Read the model definition and answer for the solid it produces. Units are mm, in the model's axes. Face numbers are marked on the shaded views. A direction names the side the tool comes from. Coordinates: 2 decimals unless noted, no trailing zeros. Loops run counter-clockwise (first coordinate to the right, second up) from the corner with the lowest first, then second, coordinate; pieces in that order, holes last.
Q1. Section D-D (z = 68) is taken. Give the vertices of the cut face in (x, y), then the cut area to 3 significant figures.
Q2. The mould has two halves that part along X. Classify the marked faces 1, 2, 3 and 4: pulls with the +X half, pulls with the -X half, needs draft (parallel to the pull), parting line crosses it, or undercut.
Q3. Section A-A (z = -12) is taken. Give the vertices of the cut face in (x, y).
Q4. Straight lines are drawn through the part: line 1 (X direction, y = 79, z = 135.5); line 2 (Y direction, x = 197.5, z = 175.5); line 3 (X direction, y = 161, z = 106). For each, find the intervals that lie inside material, in ascending order.
Q5. Section C-C (x = 156) is taken. Give the vertices of the cut face in (y, z).
Q6. Section B-B (y = 369) is taken. Give the vertices of the cut face in (x, z).
Q7. Which of the six approach directions +Z, -Z, +X, -X, +Y, -Y give full straight-line access (tool end or side, diameter ignored) to the marked faces 5, 6 and 7?
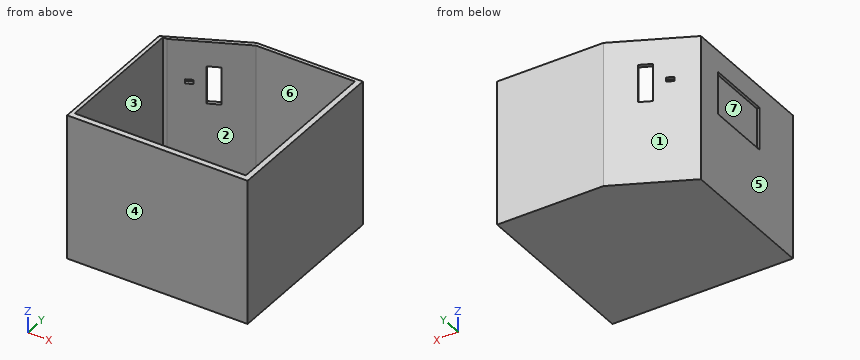
from build123d import *

# Parameters (mm, degrees)
SKETCH1_W           = 508
SKETCH1_H           = 408
SKETCH1_W_2         = 500
SKETCH1_H_2         = 400
BOSS_EXTRUDE1_DEPTH = 500
SKETCH1_3_W         = 500
SKETCH1_3_H         = 400
BOSS_EXTRUDE2_DEPTH = 500
SKETCH2_W           = 120
SKETCH2_H           = 180
CUT_EXTRUDE1_DEPTH  = 7.5
SKETCH4_W           = 481.787571452
SKETCH4_H           = 382.410311639
CUT_EXTRUDE3_DEPTH  = 404
CUT_EXTRUDE4_DEPTH  = 434
CUT_EXTRUDE5_DEPTH  = 404
SKETCH10_W          = 20
SKETCH10_H          = 12
SKETCH10_W_2        = 35.5
SKETCH10_H_2        = 106
CUT_EXTRUDE6_DEPTH  = 24


with BuildPart() as part:
    # Sketch1 → Boss-Extrude1 (new body)
    with BuildSketch(Plane(origin=(0, 0, 0), x_dir=(1, 0, 0), z_dir=(0, 1, 0))):
        with Locations((-0.117405467, -0.781547842)):
            Rectangle(SKETCH1_W, SKETCH1_H)
        with Locations((-0.117405467, -0.781547842)):
            Rectangle(SKETCH1_W_2, SKETCH1_H_2, mode=Mode.SUBTRACT)
    extrude(amount=BOSS_EXTRUDE1_DEPTH)

    # Sketch1_3 → Boss-Extrude2 (add)
    with BuildSketch(Plane(origin=(0, 0, 0), x_dir=(1, 0, 0), z_dir=(0, 1, 0))):
        with Locations((-0.117405467, -0.781547842)):
            Rectangle(SKETCH1_3_W, SKETCH1_3_H)
    extrude(amount=BOSS_EXTRUDE2_DEPTH)

    # Sketch2 → Cut-Extrude1 (cut, symmetric)
    with BuildSketch(Plane.ZY.offset(254.117405467)):
        with Locations((84.712563528, 234.953187265)):
            Rectangle(SKETCH2_W, SKETCH2_H)
    extrude(amount=CUT_EXTRUDE1_DEPTH, both=True, mode=Mode.SUBTRACT)

    # Sketch4 → Cut-Extrude3 (cut, symmetric)
    with BuildSketch(Plane.XY.offset(204.781547842)):
        with Locations((-2.789371367, 207.878900207)):
            Rectangle(SKETCH4_W, SKETCH4_H)
    extrude(amount=CUT_EXTRUDE3_DEPTH, both=True, mode=Mode.SUBTRACT)

    # Sketch8 → Cut-Extrude4 (cut, symmetric)
    with BuildSketch(Plane.XY.offset(204.781547842)):
        Polygon((-254.117405467, 399.203948512), (-253.994172888, 399.203948512), (-45.39037666, 500), (-254.117405467, 500), align=None)
    extrude(amount=CUT_EXTRUDE4_DEPTH, both=True, mode=Mode.SUBTRACT)

    # Sketch9 → Cut-Extrude5 (cut, symmetric)
    with BuildSketch(Plane.XY.offset(204.781547842)):
        Polygon((-40.587805706, 489.7694832), (-231.625791255, 399.084056026), (238.104414359, 399.084056026), (238.104414359, 398.17698413), (238.202409937, 398.17698413), (238.202409937, 489.7694832), align=None)
    extrude(amount=CUT_EXTRUDE5_DEPTH, both=True, mode=Mode.SUBTRACT)

    # Sketch10 → Cut-Extrude6 (cut, symmetric)
    with BuildSketch(Plane(origin=(-204.45830182, 423.139372032, 0), x_dir=(0.900398188, 0.435066781, 0), z_dir=(-0.435066781, 0.900398188, 0))):
        with Locations((17.482156961, -87.755377662)):
            Rectangle(SKETCH10_W, SKETCH10_H)
        with Locations((77.005207248, -82.022659024)):
            Rectangle(SKETCH10_W_2, SKETCH10_H_2)
    extrude(amount=CUT_EXTRUDE6_DEPTH, both=True, mode=Mode.SUBTRACT)


solid = part.part
Numbers:
1. outline: (-254.12, 0) - (253.88, 0) - (253.88, 500) - (-45.39, 500) - (-119.14, 464.36) - (-114.47, 454.7) - (-40.59, 489.77) - (238.2, 489.77) - (238.2, 398.18) - (238.1, 398.18) - (238.1, 16.67) - (-243.68, 16.67) - (-243.68, 399.08) - (-231.63, 399.08) - (-146.54, 439.47) - (-151.11, 448.92) - (-253.99, 399.2) - (-254.12, 399.2) - (-254.12, 324.95) - (-246.62, 324.95) - (-246.62, 144.95) - (-254.12, 144.95) - close
1. area: 23,600 mm2
2. face 1: pulls with the -X half
2. face 2: undercut
2. face 3: undercut
2. face 4: needs draft
3. outline: (-254.12, 0) - (253.88, 0) - (253.88, 500) - (-45.39, 500) - (-253.99, 399.2) - (-254.12, 399.2) - close; hole (-243.68, 16.67) - (238.1, 16.67) - (238.1, 398.18) - (238.2, 398.18) - (238.2, 489.77) - (-40.59, 489.77) - (-231.63, 399.08) - (-243.68, 399.08) - close
4. line 1: x = -254.12 to -243.68, 238.1 to 253.88
4. line 2: y = 0 to 16.67, 489.77 to 500
4. line 3: x = -246.62 to -243.68, 238.1 to 253.88
5. outline: (0, -203.22) - (500, -203.22) - (500, 204.78) - (489.77, 204.78) - (489.77, -199.22) - (16.67, -199.22) - (16.67, 204.78) - (0, 204.78) - close
6. outline: (-254.12, -203.22) - (253.88, -203.22) - (253.88, 204.78) - (238.1, 204.78) - (238.1, -199.22) - (-243.68, -199.22) - (-243.68, 204.78) - (-254.12, 204.78) - close
7. face 5: +Z, -Z, -X, +Y, -Y
7. face 6: +Z
7. face 7: -X
